```python
from build123d import *

# Parameters (mm, degrees)
F0_W     = 180
F0_H     = 30
F0_R     = 2.5751263091
F1_DEPTH = 4
F2_R     = 1
F3_R     = 0.5


# Not quite as in the source:
# - a feature names something its author has since deleted; it is built from what else it names


with BuildPart() as f1:
    # F0 (on Front) → F1 (new body)
    with BuildSketch(Plane.XZ):
        Rectangle(F0_W, F0_H)
        with Locations((-85, -10)):
            Circle(F0_R, mode=Mode.SUBTRACT)
        with Locations((85, -10)):
            Circle(F0_R, mode=Mode.SUBTRACT)
        with Locations((-85, 10)):
            Circle(F0_R, mode=Mode.SUBTRACT)
        with Locations((85, 10)):
            Circle(F0_R, mode=Mode.SUBTRACT)
    extrude(amount=F1_DEPTH)

    # F2
    f2_edges = [f1.edges().sort_by_distance(p)[0] for p in [
        (-87.575126, -4, 10),
        (-87.575126, -4, -10),
        (82.424874, -4, 10),
        (82.424874, -4, -10),
    ]]
    fillet(f2_edges, radius=F2_R)

    # F3
    f3_edges = [f1.edges().sort_by_distance(p)[0] for p in [
        (0, -4, 15),
        (-90, -4, 0),
        (0, -4, -15),
        (90, -4, 0),
        (-90, -2, 15),
        (-90, -2, -15),
        (90, -2, 15),
        (90, -2, -15),
    ]]
    fillet(f3_edges, radius=F3_R)


solid = f1.part
```
Input: part model. Units: mm. Frame: model coordinates. Coordinates: 2 decimals unless noted, no trailing zeros. Write each loop counter-clockwise with the first axis right and the second up, starting at its lowest first coordinate (ties: lowest second). Pieces come first, ordered by that corner, then holes.
1) Pin query (flat end, axial travel): pin 1 Ø4 at (x, z) = (-85, -10) entering from +Y; pin 2 Ø6.5 at (x, z) = (85, 10) entering from -Y. Return the tip coordinate at first contact, or that it passes through.
2) Section B-B on z = 10. Output: boundary loops of the cut face in (x, y).
3) Section A-A on x = 85. Output: boundary loops of the cut face in (y, z).
4) Material intervals for line 1 along Z through (x, y) = (85, -1.65); line 2 along X through (y, z) = (-0.25, 7.75); line 3 along X through (y, z) = (-1.7, -10.75), sorted ascending.
5) Section C-C on y = -2.4. Output: boundary loops of the cut face in (x, z).
6) Mould query, pull axis X, two halves, no side actions, for faces 1 (the flat face through (-90, -2, 0)), 2 (the flat face through (-1, -4, 0)), 3 (the cylindrical face through (-82.544, -1.479, -9.227)). Classes: pulls with the +X half, pulls with the -X half, needs draft (parallel to the pull), parting line crosses it, or undercut.
Check result:
1. pin 1: passes through
1. pin 2: stops at y = -3.95
2. outline: (-90, -3.5) arc R0.5 ccw to (-89.5, -4) - (-88.58, -4) arc R1 ccw to (-87.58, -3) - (-87.58, 0) - (-90, 0) - close; (-82.42, -3) arc R1 ccw to (-81.42, -4) - (81.42, -4) arc R1 ccw to (82.42, -3) - (82.42, 0) - (-82.42, 0) - close; (87.58, -3) arc R1 ccw to (88.58, -4) - (89.5, -4) arc R0.5 ccw to (90, -3.5) - (90, 0) - (87.58, 0) - close
3. outline: (-4, -14.5) arc R0.5 ccw to (-3.5, -15) - (0, -15) - (0, -12.58) - (-3, -12.58) arc R1 ccw to (-4, -13.58) - close; (-4, -6.42) arc R1 ccw to (-3, -7.42) - (0, -7.42) - (0, 7.42) - (-3, 7.42) arc R1 ccw to (-4, 6.42) - close; (-4, 13.58) arc R1 ccw to (-3, 12.58) - (0, 12.58) - (0, 15) - (-3.5, 15) arc R0.5 ccw to (-4, 14.5) - close
4. line 1: z = -15 to -12.58, -7.42 to 7.42, 12.58 to 15
4. line 2: x = -90 to -86.25, -83.75 to 83.75, 86.25 to 90
4. line 3: x = -90 to -87.46, -82.54 to 82.54, 87.46 to 90
5. outline: (-90, -14.5) arc R0.5 ccw to (-89.5, -15) - (89.5, -15) arc R0.5 ccw to (90, -14.5) - (90, 14.5) arc R0.5 ccw to (89.5, 15) - (-89.5, 15) arc R0.5 ccw to (-90, 14.5) - close; hole circle Ø5.15 at (-85, -10); hole circle Ø5.15 at (-85, 10); hole circle Ø5.15 at (85, -10); hole circle Ø5.15 at (85, 10)
6. face 1: pulls with the -X half
6. face 2: needs draft
6. face 3: undercut
